The figure shows three views and two pictorial views of one solid part (mm, origin at its lowest corner). Answer the questions. Round coordinates to 2 decimals unless told otherwise and drop trailing zeros. Loops run counter-clockwise (first coordinate to the right, second up) from the corner with the lowest first, then second, coordinate; pieces in that order, holes last. Notation, with made-up numbers: (57, 29) -> (77, 29) arc R18 cw to (77, 33) -> close; hole circle Ø6 at (62, 77.5). An arc over 180 degrees is marked (long way). Write each question's results on one line, items separated by ' | '. Start each with the question number.
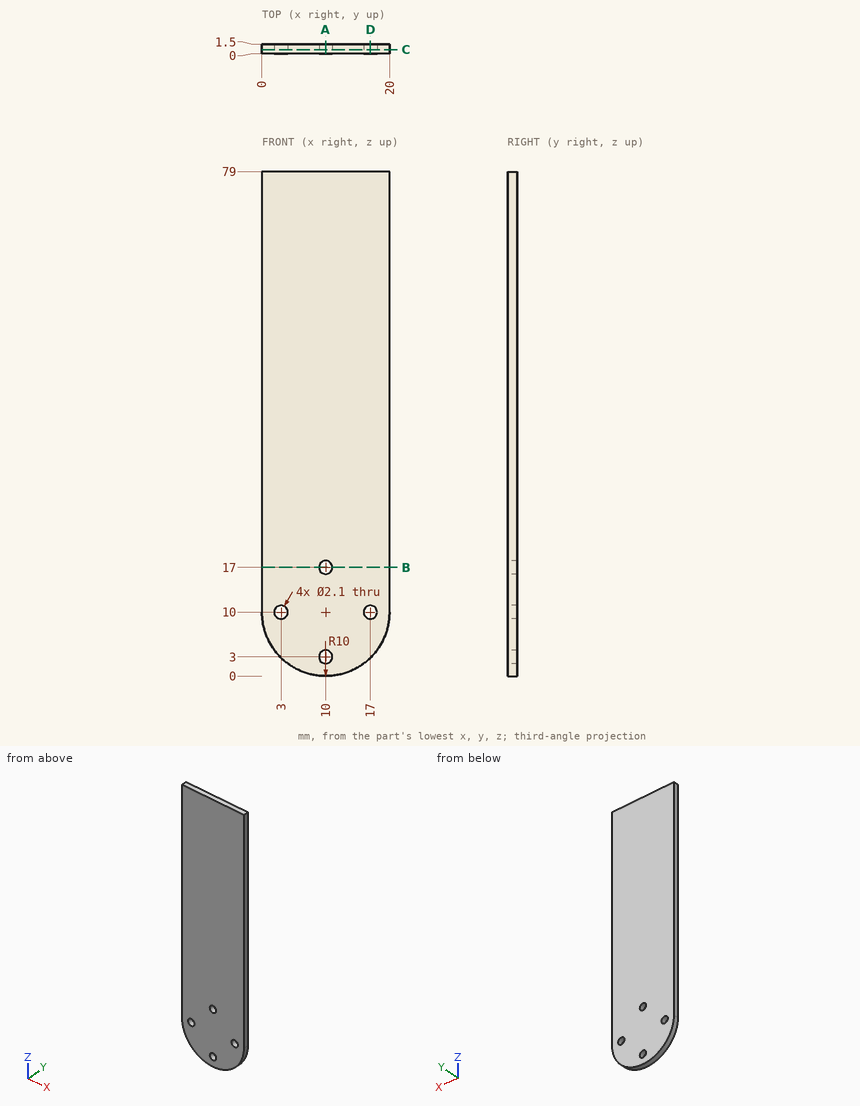
Item 1: Straight lines are drawn through the part: L1, parallel to Z at x = 10, y = 0.35; L2, parallel to X at y = 0.9, z = 10; L3, parallel to X at y = 0.45, z = 3. For each, find the intervals that lie inside material, in ascending order. Write a range as [from, to].
Item 2: The part is cut by section C-C, the plane y = 0.6. Give the vertices of the cut face in (x, z), plus the area to 3 significant figures.
Item 3: The part is cut by section A-A, the plane x = 10. Give the vertices of the cut face in (y, z).
Item 4: The part is cut by section B-B, the plane z = 17. Give the vertices of the cut face in (x, y).
Item 5: The part is cut by section D-D, the plane x = 17. Give the vertices of the cut face in (y, z), plus the area to 3 significant figures.
Item 6: This flat-tipped pin is pushed along its axis until it touches: pin 1 Ø1.9 at (x, z) = (10, 3) entering from +Y. Where does it stop, or does it pass through?
Report:
1) L1: z = [0, 1.95], [4.05, 15.95], [18.05, 79] | L2: x = [0, 1.95], [4.05, 15.95], [18.05, 20] | L3: x = [2.86, 8.95], [11.05, 17.14]
2) outline: (0, 10) arc R10 ccw to (20, 10) -> (20, 79) -> (0, 79) -> close; hole circle Ø2.1 at (3, 10); hole circle Ø2.1 at (10, 3); hole circle Ø2.1 at (10, 17); hole circle Ø2.1 at (17, 10) | area: 1,520 mm2
3) outline: (0, 0) -> (1.5, 0) -> (1.5, 1.95) -> (0, 1.95) -> close; (0, 4.05) -> (1.5, 4.05) -> (1.5, 15.95) -> (0, 15.95) -> close; (0, 18.05) -> (1.5, 18.05) -> (1.5, 79) -> (0, 79) -> close
4) outline: (0, 0) -> (8.95, 0) -> (8.95, 1.5) -> (0, 1.5) -> close; (11.05, 0) -> (20, 0) -> (20, 1.5) -> (11.05, 1.5) -> close
5) outline: (0, 2.86) -> (1.5, 2.86) -> (1.5, 8.95) -> (0, 8.95) -> close; (0, 11.05) -> (1.5, 11.05) -> (1.5, 79) -> (0, 79) -> close | area: 111 mm2
6) pin 1: passes through
